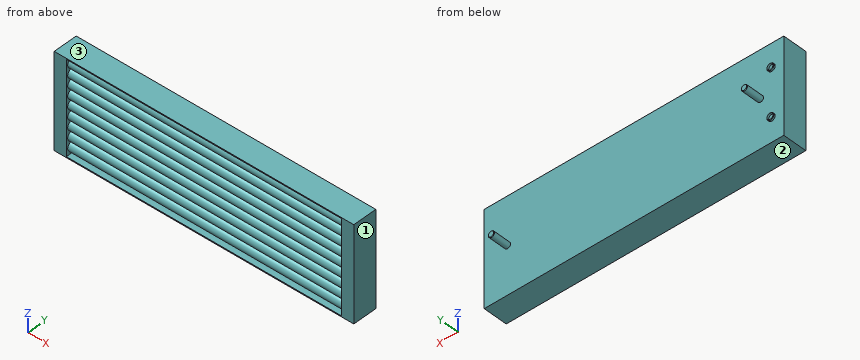
Autodesk Inventor part; units mm, degrees
ref_plane "YZ Plane" through (0, 0, 0) normal (1, 0, 0) x (0, 1, 0)
ref_plane "XZ Plane" through (0, 0, 0) normal (0, 1, 0) x (-1, 0, 0)
ref_plane "XY Plane" through (0, 0, 0) normal (0, 0, 1) x (1, 0, 0)
sketch "Boceto1" plane through (0, 0, 0) normal (0, 1, 0) x (-1, 0, 0)
  line L0 (-157.5, 50) -> (157.5, 50)
  line L1 (157.5, 50) -> (157.5, -50)
  line L2 (157.5, -50) -> (-157.5, -50)
  line L3 (-157.5, -50) -> (-157.5, 50)
  line L4 (-157.5, 50) -> (157.5, -50) construction
  line L5 (157.5, 50) -> (-157.5, -50) construction
  point P0 (0, 0)
  dimension "d0" = 315
  dimension "d1" = 100
extrude "Extrusión1" add sketch "Boceto1" along normal blind 25.4
sketch "Boceto2" plane through (0, 0, 0) normal (0, -1, 0) x (1, 0, 0)
  line L0 (-144.8, 48.98) -> (144.8, 48.98)
  line L1 (144.8, -48.98) -> (-144.8, -48.98)
  line L2 (-144.8, -48.98) -> (-144.8, 48.98)
  line L3 (144.8, 48.98) -> (144.8, -48.98)
  line L4 (-157.5, -50) -> (-157.5, 50)
  line L5 (-157.5, 50) -> (157.5, 50)
  line L6 (157.5, 50) -> (157.5, -50)
  dimension "d8" = 12.7
  dimension "d9" = 1.02
  dimension "d52" = 12.7
extrude "Extrusión2" cut sketch "Boceto2" against normal blind 24.38
sketch "Boceto4" plane through (0, 25.4, 0) normal (0, 1, 0) x (1, 0, 0)
  line L0 (-157.5, 50) -> (-108.5, 50) construction
  line L1 (-108.5, 50) -> (-108.5, -50) construction
  line L2 (-157.5, -50) -> (157.5, -50) construction
  line L3 (-157.5, -50) -> (-108.5, 50) construction
  line L4 (-157.5, 50) -> (-108.5, -50) construction
  line L5 (157.5, 50) -> (-157.5, 50) construction
  line L6 (157.5, 50) -> (108.5, 50) construction
  line L7 (108.5, 50) -> (108.5, -50) construction
  line L8 (108.5, -50) -> (157.5, 50) construction
  line L9 (108.5, 50) -> (157.5, -50) construction
  circle A0 centre (-133, 0) radius 3.175
  circle A1 centre (133, 0) radius 3.175
  point P0 (0, 0)
  dimension "d24" = 49
  dimension "d25" = 49
  dimension "d26" = 6.35
  dimension "d27" = 6.35
extrude "Extrusión4" add sketch "Boceto4" along normal blind 19.05
thread "Rosca1"
thread "Rosca2"
chamfer "Chaflán1" distance 0.5 angle 45 1 edges at (-136.175, 44.45, 0)
chamfer "Chaflán2" distance 0.5 angle 45 1 edges at (129.825, 44.45, 0)
sketch "Boceto6" plane through (-144.8, 0, 48.98) normal (1, 0, 0) x (0, 0, -1)
  circle A0 centre (7, 6.35) radius 4.7625
  line L0 (0, 0) -> (0, 24.38)
  line L1 (97.96, 0) -> (0, 0)
  circle A1 centre (17.5, 6.35) radius 4.7625
  circle A2 centre (28, 6.35) radius 4.7625
  circle A3 centre (38.5, 6.35) radius 4.7625
  circle A4 centre (49, 6.35) radius 4.7625
  circle A5 centre (59.5, 6.35) radius 4.7625
  circle A6 centre (70, 6.35) radius 4.7625
  circle A7 centre (80.5, 6.35) radius 4.7625
  circle A8 centre (91, 6.35) radius 4.7625
  point P0 (48.98, 0)
  dimension "d53" = 9.525
  dimension "d54" = 7
  dimension "d55" = 6.35
  dimension "d58" = 10.5
extrude "Extrusión6" add sketch "Boceto6" along normal up to surface (289.6 mm away)
sketch "Boceto7" plane through (0, 25.4, 0) normal (0, 1, 0) x (1, 0, 0)
  line L0 (-157.5, 50) -> (-157.5, -50) construction
  line L1 (-157.5, 0) -> (-144.8, 0) construction
  line L2 (-144.8, 0) -> (-144.8, 25) construction
  line L3 (-144.8, 48.98) -> (-144.8, -48.98) construction
  line L4 (-144.8, 0) -> (-144.8, -25) construction
  circle A0 centre (-144.8, -25) radius 3.175
  circle A1 centre (-144.8, 25) radius 3.175
  circle A2 centre (-144.8, -25) radius 3.685
  circle A3 centre (-144.8, 25) radius 3.685
  point P0 (0, 0)
  dimension "d67" = 12.7
  dimension "d68" = 25
  dimension "d69" = 25
  dimension "d70" = 6.35
  dimension "d71" = 6.35
  dimension "d72" = 7.37
  dimension "d73" = 7.37
extrude "Extrusión7" add sketch "Boceto7" along normal blind 2
chamfer "Chaflán4" distance 0.5 angle 45 2 edges at (-148.485, 27.4, 25) (-148.485, 27.4, -25)
sketch "Boceto8" plane through (-144.8, 25.4, -25) normal (0, 1, 0) x (1, 0, 0)
  circle A0 centre (0, 0) radius 3.175
sketch "Boceto9" plane through (-144.8, 25.4, 25) normal (0, 1, 0) x (1, 0, 0)
  circle A0 centre (0, 0) radius 3.175
properties part number "resistencia_cuarzo_550W"
Check sheet for the modelled part. Datum: model origin and axes. Units: mm. Face numbers are marked on the shaded views. Give positions to 0.01 mm unless a question says otherwise; leave off trailing zeros. Loops run counter-clockwise (first coordinate to the right, second up) from the corner with the lowest first, then second, coordinate; pieces in that order, holes last. Notation, with made-up numbers: M 31,89.5 L 74,89.5 A28 ccw 74,127.5 Z; hole C -13,73.5 d6. An arc over 180 degrees is marked long. Answer in a Markdown table with one row per item.
1) Cross-section at A-A (y = 21). Enter the section's corners in (x, z), plus the area to 3 significant figures.
Solutions:
| item | result |
|---|---|
| outline | M -157.5,-50 L 157.5,-50 L 157.5,50 L -157.5,50 Z; hole M -144.8,-48.98 L 144.8,-48.98 L 144.8,48.98 L -144.8,48.98 Z |
| area | 3,130 mm^2 |
2) Cross-section at B-B (x = 125.5). Count the separate pieces of the cut face and the enclosed holes in it, plus the area to 3 significant figures.
Solutions:
| item | result |
|---|---|
| separate pieces | 10 |
| enclosed holes | 0 |
| area | 793 mm^2 |
3) Depth check by flat-ended pin: pin 1 (8 mm diameter, centred on x = -25, z = -27.5, fed in from +Y); pin 2 (5 mm diameter, centred on x = -145, z = -23.5, fed in from +Y); pin 3 (3 mm diameter, centred on y = 35, z = -1, fed in from +X) (3 decimals); pin 4 (4 mm diameter, centred on y = 30.5, z = -7, fed in from -X). Enter the tip coordinate at first touch or a pass-through.
Solutions:
| item | result |
|---|---|
| pin 1 | stops at y = 25.4 |
| pin 2 | stops at y = 27.4 |
| pin 3 | stops at x = 136.175 |
| pin 4 | passes through |
4) Cross-section at C-C (z = -10.52). Enter the section's corners in (x, y).
Solutions:
| item | result |
|---|---|
| outline | M -157.5,0 L -144.8,0 L -144.8,1.59 L 144.8,1.59 L 144.8,0 L 157.5,0 L 157.5,25.4 L -157.5,25.4 Z; hole M -144.8,11.11 L 144.8,11.11 L 144.8,24.38 L -144.8,24.38 Z |
5) Thickness scan on line 1 (Z direction, x = -144.8, y = 26.7) (3 decimals); line 2 (X direction, y = 20, z = -43); line 3 (Z direction, x = -144, y = 26). Record the ranges inside material, lowest first.
Solutions:
| item | result |
|---|---|
| line 1 | z = -28.685 to -28.175, -21.825 to -21.315, 21.315 to 21.825, 28.175 to 28.685 |
| line 2 | x = -157.5 to -144.8, 144.8 to 157.5 |
| line 3 | z = -28.6 to -28.07, -21.93 to -21.4, 21.4 to 21.93, 28.07 to 28.6 |
6) Mould release check, pull along Z, two halves, no side actions. Record for the marked faces 1, 2 and 3: released by +Z, released by -Z, zero draft, split by the parting line, or undercut.
Solutions:
| item | result |
|---|---|
| face 1 | zero draft |
| face 2 | released by -Z |
| face 3 | released by +Z |
